For this review, take the finished solid that the model builds, in its own axes (mm). A direction names the side the tool comes from. Coordinates: 2 decimals unless noted, no trailing zeros. Order: outer loops, then holes, each group sorted by start corner. A loop starts at its lowest first (then second) coordinate and runs counter-clockwise, first axis right, second up. Notation, with made-up numbers: (-1, 20.25) -> (49, 20.25) arc R38 cw to (49, 58.25) -> close; hole circle Ø4 at (44.25, 38.5). An arc over 180 degrees is marked (long way). Answer as a JSON object with one key per item and string values. Group by question number.
1) Add section D-D, the plane x = 12. Write out the cut boundary in (y, z), then the cut area to 3 significant figures.
2) Add section C-C, the plane y = 0. Write out the cut boundary in (x, z).
3) Add section A-A, the plane z = 14. Write out the cut boundary in (x, y), then the cut area to 3 significant figures.
4) Add section B-B, the plane x = 0. Write out the cut boundary in (y, z).
5) Wall thickness on L1, parallel to Y at x = 0, z = 17.75; L2, parallel to X at y = 38.5, z = 20; L3, parallel to Z at x = 10.5, y = 36.5: over which ranges is each line inside the solid? List them lowest first.
6) For pin 1 (2.5 mm diameter, centred on x = 12, z = 5, fed in from +Y); pin 2 (1.2 mm diameter, centred on x = 12.5, z = 5.5, fed in from -Y), all flat-tipped, find the tip position at first contact; note any pin that passes through.
7) Machinability: for faces 1 (the cylindrical face through (-2.21, 32.03, 12.32)), 2 (the cylindrical face through (13.352, -36.675, 3.526)), 3 (the flat face through (12, 24, 5)), which of the approach directions +Z, -Z, +X, -X, +Y, -Y give a long, thin tool a straight path to every point of the face, cutting with its end or side? Answer none if there is none.
8) Draft analysis for pull direction X (two halves, no side actions). For faces 4 (the flat face through (-10, -1, 12)), 5 (the flat face through (6, 1, 25)), 6 (the cylindrical face through (14, 37, 20)), state which applies: +X half, -X half, draft (parallel to the pull), parting line (faces both ways), or undercut.
from build123d import *

# Parameters (mm, degrees)
SKETCH1_W           = 20
SKETCH1_H           = 98
SKETCH1_R           = 4
SKETCH1_R_2         = 3
BOSS_EXTRUDE1_DEPTH = 25
SKETCH2_W           = 11
SKETCH2_H           = 98
BOSS_EXTRUDE2_DEPTH = 25
SKETCH3_R           = 2
CUT_EXTRUDE1_DEPTH  = 25


with BuildPart() as part:
    # Sketch1 → Boss-Extrude1 (new body)
    with BuildSketch(Plane.XY):
        Rectangle(SKETCH1_W, SKETCH1_H)
        Circle(SKETCH1_R, mode=Mode.SUBTRACT)
        with Locations((0, -30)):
            Circle(SKETCH1_R_2, mode=Mode.SUBTRACT)
        with Locations((0, 30)):
            Circle(SKETCH1_R_2, mode=Mode.SUBTRACT)
    extrude(amount=BOSS_EXTRUDE1_DEPTH)

    # Sketch2 → Boss-Extrude2 (add, through all)
    with BuildSketch(Plane(origin=(0, 0, 0), x_dir=(-1, 0, 0), z_dir=(0, 0, -1))):
        with Locations((-15.5, 0)):
            Rectangle(SKETCH2_W, SKETCH2_H)
    extrude(amount=-BOSS_EXTRUDE2_DEPTH)

    # Sketch3 → Cut-Extrude1 (cut)
    with BuildSketch(Plane(origin=(0, 49, 0), x_dir=(1, 0, 0), z_dir=(0, 1, 0))):
        with Locations(Location((12, -5, 0), (0, 0, 270))):
            Circle(SKETCH3_R)
        with Locations(Location((12, -20, 0), (0, 0, 270))):
            Circle(SKETCH3_R)
    cut_extrude1 = extrude(amount=-CUT_EXTRUDE1_DEPTH, mode=Mode.SUBTRACT)

    # Mirror1: Cut-Extrude1 across plane
    add(cut_extrude1.mirror(Plane.ZX), mode=Mode.SUBTRACT)


solid = part.part
Output values:
{
 "1": {"outline": "(-49, 0) -> (49, 0) -> (49, 3) -> (24, 3) -> (24, 7) -> (49, 7) -> (49, 18) -> (24, 18) -> (24, 22) -> (49, 22) -> (49, 25) -> (-49, 25) -> (-49, 22) -> (-24, 22) -> (-24, 18) -> (-49, 18) -> (-49, 7) -> (-24, 7) -> (-24, 3) -> (-49, 3) -> close", "area": "2,050 mm²"},
 "2": {"outline": "(-10, 0) -> (-4, 0) -> (-4, 25) -> (-10, 25) -> close; (4, 0) -> (21, 0) -> (21, 25) -> (4, 25) -> close"},
 "3": {"outline": "(-10, -49) -> (21, -49) -> (21, 49) -> (-10, 49) -> close; hole circle Ø8 at (0, 0); hole circle Ø6 at (0, -30); hole circle Ø6 at (0, 30)", "area": "2,930 mm²"},
 "4": {"outline": "(-49, 0) -> (-33, 0) -> (-33, 25) -> (-49, 25) -> close; (-27, 0) -> (-4, 0) -> (-4, 25) -> (-27, 25) -> close; (4, 0) -> (27, 0) -> (27, 25) -> (4, 25) -> close; (33, 0) -> (49, 0) -> (49, 25) -> (33, 25) -> close"},
 "5": {"L1": "y = -49 to -33, -27 to -4, 4 to 27, 33 to 49", "L2": "x = -10 to 10, 14 to 21", "L3": "z = 0 to 3.68, 6.32 to 18.68, 21.32 to 25"},
 "6": {"pin 1": "stops at y = 24", "pin 2": "stops at y = -24"},
 "7": {"face 1": "+Z, -Z", "face 2": "-Y", "face 3": "+Y"},
 "8": {"face 4": "-X half", "face 5": "draft", "face 6": "undercut"}
}
